```python
from build123d import *

# Parameters (mm, degrees)
SKETCH_3_W               = 15.8
SKETCH_3_H               = 25
EXTRUDE_2_DEPTH          = 35
SKETCH_4_R               = 5.25
SKETCH_4_R_2             = 4.25
CUT_EXTRUDE_1_DEPTH      = 10
CUT_EXTRUDE_3_DEPTH      = 38.995526052
CUT_EXTRUDE_3_DEPTH_BACK = 38.995526052
FILLET_1_R               = 2
CHAMFER_1_SIZE           = 1


with BuildPart() as part:
    # 스케치3 → 보스-돌출2 (new body)
    with BuildSketch(Plane.XY):
        Rectangle(SKETCH_3_W, SKETCH_3_H)
    extrude(amount=EXTRUDE_2_DEPTH)

    # 스케치4 → 컷-돌출1 (cut)
    with BuildSketch(Plane.XY.offset(35)):
        Circle(SKETCH_4_R)
        Circle(SKETCH_4_R_2, mode=Mode.SUBTRACT)
    extrude(amount=-CUT_EXTRUDE_1_DEPTH, mode=Mode.SUBTRACT)

    # 스케치5 → 컷-돌출3 (cut, two sides: drawn at the far end of the back side and taken through both)
    with BuildSketch(Plane(origin=(0, 0, 0), x_dir=(0, 0, -1), z_dir=(1, 0, 0)).offset(-CUT_EXTRUDE_3_DEPTH_BACK)):
        Polygon((2.109074987, 6.770011202), (-5, 6.004306325), (-5, -6.004306325), (2.109074987, -6.770011202), align=None)
    extrude(amount=CUT_EXTRUDE_3_DEPTH + CUT_EXTRUDE_3_DEPTH_BACK, mode=Mode.SUBTRACT)

    # 필렛1
    fillet_1_edges = [part.edges().sort_by_distance(p)[0] for p in [
        (-4.25, 0, 35),
    ]]
    fillet(fillet_1_edges, radius=FILLET_1_R)

    # 모따기1
    chamfer_1_edges = [part.edges().sort_by_distance(p)[0] for p in [
        (-7.9, 0, 35),
        (0, -12.5, 35),
        (7.9, 9.521423383, 0),
        (-7.9, -9.521423383, 0),
        (7.9, 0, 35),
        (0, -12.5, 0),
        (-7.9, 9.521423383, 0),
        (0, 12.5, 0),
        (7.9, -9.521423383, 0),
        (0, 12.5, 35),
        (7.9, -12.5, 17.5),
        (-7.9, -12.5, 17.5),
        (-7.9, 12.5, 17.5),
        (7.9, 12.5, 17.5),
    ]]
    chamfer(chamfer_1_edges, length=CHAMFER_1_SIZE)


solid = part.part
```
Design review of the part built by this model. Coordinates are the model's own, in mm. Give positions to 0.01 mm unless a question says otherwise; leave off trailing zeros. Write each loop counter-clockwise with the first axis right and the second up, starting at its lowest first coordinate (ties: lowest second). Pieces come first, ordered by that corner, then holes.
(1) Add section A-A (z = 30). Give the boundary of the cut face in (x, y), and give its area (3 significant figures).
Checked values:
outline: (-7.9, -11.5) - (-6.9, -12.5) - (6.9, -12.5) - (7.9, -11.5) - (7.9, 11.5) - (6.9, 12.5) - (-6.9, 12.5) - (-7.9, 11.5) - close; circle Ø8.5 at (0, 0); hole circle Ø10.5 at (0, 0)
area: 363 mm2
(2) Mouldability with a two-part tool opening along Y and no side actions: class faces 1 (the face through (-7.9, 0, 17)), 2 (the face through (-0.11, -6.27, 2.53)), 3 (the face through (7.3, -11.8, 0.7)), 4 (the face through (0, 0, 5)) as +Y half, -Y half, draft (parallel to the pull), parting line (faces both ways), or undercut.
Checked values:
face 1: draft
face 2: undercut
face 3: -Y half
face 4: undercut
(3) Add section B-B (y = 0). Give the boundary of the cut face in (x, z), and give its area (3 significant figures).
Checked values:
outline: (-7.9, 5) - (7.9, 5) - (7.9, 34) - (6.9, 35) - (5.25, 35) - (5.25, 25) - (4.25, 25) - (4.25, 33) arc R2 ccw to (2.25, 35) - (-2.25, 35) arc R2 ccw to (-4.25, 33) - (-4.25, 25) - (-5.25, 25) - (-5.25, 35) - (-6.9, 35) - (-7.9, 34) - close
area: 451 mm2
(4) Add section D-D (z = 3.5). Give the boundary of the cut face in (x, y), and give its area (3 significant figures).
Checked values:
outline: (-7.9, -11.5) - (-6.9, -12.5) - (6.9, -12.5) - (7.9, -11.5) - (7.9, -6.17) - (-7.9, -6.17) - close; (-7.9, 6.17) - (7.9, 6.17) - (7.9, 11.5) - (6.9, 12.5) - (-6.9, 12.5) - (-7.9, 11.5) - close
area: 198 mm2
(5) Add section C-C (x = 0). Give the boundary of the cut face in (y, z).
Checked values:
outline: (-12.5, 1) - (-11.5, 0) - (-6.54, 0) - (-6, 5) - (6, 5) - (6.54, 0) - (11.5, 0) - (12.5, 1) - (12.5, 34) - (11.5, 35) - (5.25, 35) - (5.25, 25) - (4.25, 25) - (4.25, 33) arc R2 ccw to (2.25, 35) - (-2.25, 35) arc R2 ccw to (-4.25, 33) - (-4.25, 25) - (-5.25, 25) - (-5.25, 35) - (-11.5, 35) - (-12.5, 34) - close
(6) Wall thickness on line 1 along Y through (x, z) = (0, 29); line 2 along X through (y, z) = (-0.25, 26); line 3 along X through (y, z) = (3, 32): over which ranges is each line inside the solid? List them lowest first.
Checked values:
line 1: y = -12.5 to -5.25, -4.25 to 4.25, 5.25 to 12.5
line 2: x = -7.9 to -5.24, -4.24 to 4.24, 5.24 to 7.9
line 3: x = -7.9 to -4.31, -3.01 to 3.01, 4.31 to 7.9
(7) Clearance check with a flat-ended pin moving along its axis: pin 1 Ø4 at (x, y) = (-1, 2) entering from -Z. State where the tip first meets the part, or that it passes through.
Checked values:
pin 1: stops at z = 5
